For this review, take the finished solid that the model builds, in its own axes (mm). A direction names the side the tool comes from. Give positions to 0.01 mm unless a question says otherwise; leave off trailing zeros. Write each loop counter-clockwise with the first axis right and the second up, starting at its lowest first coordinate (ties: lowest second). Pieces come first, ordered by that corner, then holes. Notation, with made-up numbers: (-26, -26.75) -> (26, -26.75) arc R19 cw to (26, 8.25) -> close; hole circle Ø8 at (78.25, 43.25). An arc over 180 degrees is marked (long way). Answer as CSV lines item,"result".
```python
from build123d import *

# Parameters (mm, degrees)
SKETCH3_R           = 0.9
SKETCH3_W           = 12.417
SKETCH3_H           = 23.449530758
BOSS_EXTRUDE6_DEPTH = 6.5


with BuildPart() as part:
    # Sketch3 → Boss-Extrude6 (new body)
    with BuildSketch(Plane.XY):
        with BuildLine():
            Line((26.008786765, 76.166270115), (26.008786765, 49.799855834))
            Line((26.008786765, 49.799855834), (29.580786765, 49.799855834))
            Line((29.580786765, 49.799855834), (29.580786765, 43.649855834))
            Line((29.580786765, 43.649855834), (26.080786765, 43.649855834))
            Line((26.080786765, 43.649855834), (26.080786765, 25.249855834))
            Line((26.080786765, 25.249855834), (29.580786765, 25.249855834))
            Line((29.580786765, 25.249855834), (29.580786765, 25.206855834))
            Line((29.580786765, 25.206855834), (29.580786765, 19.279855834))
            Line((29.580786765, 19.279855834), (55.980786765, 19.279855834))
            Line((55.980786765, 19.279855834), (55.980786765, 25.249855834))
            Line((55.980786765, 25.249855834), (59.480786765, 25.249855834))
            Line((59.480786765, 25.249855834), (59.480786765, 43.649855834))
            Line((59.480786765, 43.649855834), (55.980786765, 43.649855834))
            Line((55.980786765, 43.649855834), (55.980786765, 49.799855834))
            Line((55.980786765, 49.799855834), (59.552786765, 49.799855834))
            Line((59.552786765, 49.799855834), (59.552786765, 76.166270115))
            ThreePointArc((59.552786765, 76.166270115), (53.346414701, 85.422492969), (42.780786765, 88.967097604))
            ThreePointArc((42.780786765, 88.967097604), (32.215158829, 85.422492969), (26.008786765, 76.166270115))
        make_face()
        with Locations((42.780786765, 50.712301369)):
            Circle(SKETCH3_R, mode=Mode.SUBTRACT)
        with Locations((42.780786765, 78.212301369)):
            Circle(SKETCH3_R, mode=Mode.SUBTRACT)
        with Locations((42.780786765, 64.937066748)):
            Rectangle(SKETCH3_W, SKETCH3_H, mode=Mode.SUBTRACT)
    extrude(amount=BOSS_EXTRUDE6_DEPTH)


solid = part.part
```
Q1. Add section C-C (z = 4). Write out the cut boundary in (x, y), plus the area to 3 significant figures.
Answer block:
outline,"(26.01, 49.8) -> (29.58, 49.8) -> (29.58, 43.65) -> (26.08, 43.65) -> (26.08, 25.25) -> (29.58, 25.25) -> (29.58, 19.28) -> (55.98, 19.28) -> (55.98, 25.25) -> (59.48, 25.25) -> (59.48, 43.65) -> (55.98, 43.65) -> (55.98, 49.8) -> (59.55, 49.8) -> (59.55, 76.17) arc R17.29 ccw to (42.78, 88.97) arc R17.29 ccw to (26.01, 76.17) -> close; hole (36.57, 53.21) -> (48.99, 53.21) -> (48.99, 76.66) -> (36.57, 76.66) -> close; hole circle Ø1.8 at (42.78, 50.71); hole circle Ø1.8 at (42.78, 78.21)"
area,"1,840 mm2"
Q2. Add section D-D (y = 84). Write out the cut boundary in (x, z), plus the area to 3 significant figures.
Answer block:
outline,"(30.58, 0) -> (54.99, 0) -> (54.99, 6.5) -> (30.58, 6.5) -> close"
area,"159 mm2"
Q3. To check wall thickness, follow probe 1 along Y at (x, z) = (42, 5.25); probe 2 along X at (y, z) = (69, 2.5); probe 3 along X at (y, z) = (25, 4). State the ranges of each line that lie inside material, in increasing order. Write a range as [from, to].
Answer block:
probe 1,"y = [19.28, 50.26], [51.16, 53.21], [76.66, 77.76], [78.66, 88.95]"
probe 2,"x = [26.01, 36.57], [48.99, 59.55]"
probe 3,"x = [29.58, 55.98]"
Q4. Draft analysis for pull direction Y (two halves, no side actions). For faces 1 (the cylindrical face through (53.472, 85.326, 3.204)), 2 (the flat face through (55.981, 22, 3)), 3 (the flat face through (28, 43.65, 3)), state which applies: released by +Y, released by -Y, zero draft, split by the parting line, or undercut.
Answer block:
face 1,"released by +Y"
face 2,"zero draft"
face 3,"undercut"
Q5. For faces 4 (the flat face through (28, 25.25, 3)), 5 (the flat face through (48.989, 65, 3)), 6 (the flat face through (58, 49.8, 3)), 7 (the flat face through (29.581, 47, 3)), 8 (the flat face through (59.481, 34, 3)), list the 3-axis set-ups (+Z, -Z, +X, -X, +Y, -Y) from which the entire face can be reached by the end or side of a thin tool; tool diameter is ignored.
Answer block:
face 4,"+Z, -Z, -X, -Y"
face 5,"+Z, -Z"
face 6,"+Z, -Z, +X"
face 7,"+Z, -Z, -X"
face 8,"+Z, -Z, +X, -Y"
Q6. Add section B-B (x = 48). Write out the cut boundary in (y, z), plus the area to 3 significant figures.
Answer block:
outline,"(19.28, 0) -> (53.21, 0) -> (53.21, 6.5) -> (19.28, 6.5) -> close; (76.66, 0) -> (88.19, 0) -> (88.19, 6.5) -> (76.66, 6.5) -> close"
area,"295 mm2"
Q7. Clearance check with flat-ended pins moving along their axes: pin 1 (1.1 mm diameter, centred on x = 42.78, y = 50.71, fed in from +Z); pin 2 (2 mm diameter, centred on x = 44, z = 4.5, fed in from +Y); pin 3 (1 mm diameter, centred on x = 58.5, z = 3, fed in from -Y); pin 4 (1 mm diameter, centred on x = 28.5, z = 4, fed in from +Y). State where each tip first meets the part, or that it passes through.
Answer block:
pin 1,"passes through"
pin 2,"stops at y = 88.97"
pin 3,"stops at y = 25.25"
pin 4,"stops at y = 82.22"
Q8. Add section A-A (y = 65.5). Write out the cut boundary in (x, z).
Answer block:
outline,"(26.01, 0) -> (36.57, 0) -> (36.57, 6.5) -> (26.01, 6.5) -> close; (48.99, 0) -> (59.55, 0) -> (59.55, 6.5) -> (48.99, 6.5) -> close"
